Work out the finished part from the listing and answer in its coordinate system (mm). A direction names the side the tool comes from. Give positions to 0.01 mm unless a question says otherwise; leave off trailing zeros. Order: outer loops, then holes, each group sorted by start corner. A loop starts at its lowest first (then second) coordinate and runs counter-clockwise, first axis right, second up. Notation, with made-up numbers: M -29.75,39 L 2.25,39 A25 ccw 2.25,70 Z; hole C 49,84 d1. An arc over 180 degrees is marked long. One line per item, written item: value.
from build123d import *

# Parameters (mm, degrees)
F0_W     = 92.144217
F0_H     = 81.716377
F1_DEPTH = 88.9
F3_D     = 6.35
F4_R     = 29.219742
F5_DEPTH = 100.838


with BuildPart() as f1:
    # F0 (on Front) → F1 (new body)
    with BuildSketch(Plane.XZ):
        with Locations((3.507545, -4.171138)):
            Rectangle(F0_W, F0_H)
    extrude(amount=F1_DEPTH)

    # F3 (through all)
    with Locations(Plane.XZ.offset(88.9)):
        with Locations((0, 0)):
            Hole(F3_D / 2)

    # F4 (on face) → F5 (join)
    with BuildSketch(Plane.XZ.offset(88.9)):
        Circle(F4_R)
    extrude(amount=F5_DEPTH)


solid = f1.part
(1) Section C-C, the plane y = -159 is taken. Give the vertices of the cut face in (x, z).
Findings:
outline: C 0,0 d58.44
(2) Find the intervals of material crossed by probe 1 along Z at (x, y) = (0, -52) (3 decimals); probe 2 along Y at (x, z) = (-35, -19.5); probe 3 along X at (y, z) = (-123.5, 14), in increasing order. Write a range as from..to.
Findings:
probe 1: z = -45.029..-3.175, 3.175..36.687
probe 2: y = -88.9..0
probe 3: x = -25.65..25.65
(3) Which of the six approach directions +Z, -Z, +X, -X, +Y, -Y give full straight-line access (tool end or side, diameter ignored) to faces 5 (the cylindrical face through (26.992, -138.613, -11.191)), 6 (the flat face through (3, -44, 36.687))?
Findings:
face 5: -Y
face 6: +Z, +X, -X, +Y, -Y
(4) Section A-A, the plane x = 0 is taken. Give the vertices of the cut face in (y, z) (3 decimals).
Findings:
outline: M -189.738,-29.22 L -88.9,-29.22 L -88.9,-45.029 L 0,-45.029 L 0,-3.175 L -88.9,-3.175 L -88.9,3.175 L 0,3.175 L 0,36.687 L -88.9,36.687 L -88.9,29.22 L -189.738,29.22 Z
(5) Given P1, Ø10, axis at y = -140, z = -3, coming from the -X side; P2, Ø8, axis at x = -9.5, z = -4, coming from the +Y side; P3, Ø3, axis at x = -32.5, z = -23.5, coming from the -Y side; P4, Ø10, axis at x = -4.5, y = -124.5, coming from the +Z side, each flat-ended and moving along its own axis, determine where each tip first touches the part or whether it passes through.
Findings:
P1: stops at x = -29.22
P2: stops at y = 0
P3: stops at y = -88.9
P4: stops at z = 29.22
(6) Section B-B, the plane z = 0 is taken. Give the vertices of the cut face in (x, y) (3 decimals).
Findings:
outline: M -42.565,-88.9 L -29.22,-88.9 L -29.22,-189.738 L 29.22,-189.738 L 29.22,-88.9 L 49.58,-88.9 L 49.58,0 L 3.175,0 L 3.175,-88.9 L -3.175,-88.9 L -3.175,0 L -42.565,0 Z
(7) Determine the mould class of faces 1 (the flat face through (49.58, -44, -5)), 2 (the flat face through (3, 0, -4)), 3 (the flat face through (0, -88.9, 0)), 4 (the cylindrical face through (0.69, -43.83, -3.1)) for opening direction X: pulls with the +X half, pulls with the -X half, needs draft (parallel to the pull), parting line crosses it, or undercut.
Findings:
face 1: pulls with the +X half
face 2: needs draft
face 3: undercut
face 4: undercut
(8) Section D-D, the plane x = -12 is taken. Give the vertices of the cut face in (y, z).
Findings:
outline: M -189.74,-26.64 L -88.9,-26.64 L -88.9,-45.03 L 0,-45.03 L 0,36.69 L -88.9,36.69 L -88.9,26.64 L -189.74,26.64 Z
